Could you check a few things on this model? Use its own coordinates, in mm. Face numbers are marked on the shaded views. A direction names the side the tool comes from. Coordinates: 2 decimals unless noted, no trailing zeros. Loops run counter-clockwise (first coordinate to the right, second up) from the corner with the lowest first, then second, coordinate; pieces in that order, holes last. Notation, with made-up numbers: (-10.5, 2) - (3.5, 2) arc R15 ccw to (3.5, 22) - close; hole circle Ø8 at (-39, 34). An arc over 180 degrees is marked (long way). One line per item, written item: value. Start each with the question number.
(1) If I drill on line 1 along Y through (x, z) = (0, 25.75); line 2 along Z through (x, y) = (-3.75, -5); line 3 along Z through (x, y) = (1.75, 0.5), over which ranges is the centre line in solid material (lowest first)? Write a range as from..to.
(2) If we section it at B-B on x = 0: Write out the boundary of the cut face in (y, z), then the cut area to 3 significant figures.
(3) If we section it at A-A on y = 0: Write out the boundary of the cut face in (x, z).
(4) If we mould it in two halves opening along X, with no side actions, what happens to the marked faces 1, 2 and 3? For each: pulls with the +X half, pulls with the -X half, needs draft (parallel to the pull), parting line crosses it, or undercut.
(5) I'm going to push flat-ended pins straight in: P1, Ø1.5, axis at y = 2, z = 23, coming from the -X side; P2, Ø5, axis at x = -6.5, z = 26.5, coming from the -Y side; P3, Ø4, axis at y = 0, z = 28, coming from the +X side. Where does each tip first touch, or does it pass through?
(6) On a 3-axis mill with a long thin cutter (end or side, diameter ignored), from which of +Z, -Z, +X, -X, +Y, -Y can I reach the whole of each face in a straight line? I mean the marked faces 4, 5 and 6. Say none if no direction works.
(7) If we section it at C-C on z = 5.75: Write out the boundary of the cut face in (x, y).
(8) If we section it at D-D on z = 18.75: Write out the boundary of the cut face in (x, y).
Autodesk Inventor part; units mm, degrees
ref_plane "YZ Plane" through (0, 0, 0) normal (1, 0, 0) x (0, 1, 0)
ref_plane "XZ Plane" through (0, 0, 0) normal (0, 1, 0) x (-1, 0, 0)
ref_plane "XY Plane" through (0, 0, 0) normal (0, 0, 1) x (1, 0, 0)
sketch "Sketch1" plane through (0, 0, 0) normal (0, 0, 1) x (1, 0, 0)
  circle A0 centre (0, 0) radius 9
  dimension "d0" = 18
extrude "Extrusion1" add sketch "Sketch1" along normal blind 10
chamfer "Chamfer1" distance 0.5 angle 45 1 edges at (-9, 0, 0)
sketch "Sketch2" plane through (0, 0, 0) normal (0, 0, -1) x (-1, 0, 0)
  circle A0 centre (0, 0) radius 2.75
  dimension "d6" = 5.5
extrude "Extrusion2" cut sketch "Sketch2" against normal blind 5
sketch "Sketch3" plane through (0, 0, 10) normal (0, 0, 1) x (1, 0, 0)
  circle A0 centre (0, 0) radius 5
  dimension "d9" = 10
extrude "Extrusion3" add sketch "Sketch3" along normal blind 20
sketch "Sketch4" plane through (0, 0, 30) normal (0, 0, 1) x (1, 0, 0)
  arc A0 (-1.1, -1.7889) -> (-1.1, 1.7889) centre (0, 0) ccw
  line L0 (-1.1, 1.7889) -> (-1.1, -1.7889)
  dimension "d12" = 4.2
  dimension "d13" = 1.1
extrude "Extrusion4" cut sketch "Sketch4" against normal blind 7
properties part number "MotorFlyWheel"
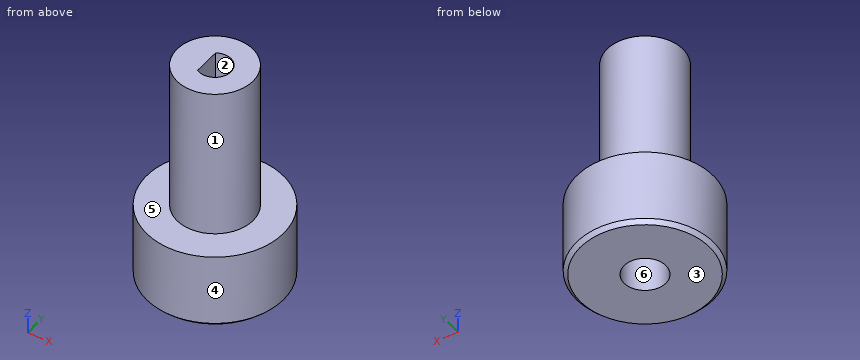
Values:
1. line 1: y = -5..-2.1, 2.1..5
1. line 2: z = 0..10
1. line 3: z = 5..23
2. outline: (-9, 0.5) - (-8.5, 0) - (-2.75, 0) - (-2.75, 5) - (2.75, 5) - (2.75, 0) - (8.5, 0) - (9, 0.5) - (9, 10) - (5, 10) - (5, 30) - (2.1, 30) - (2.1, 23) - (-2.1, 23) - (-2.1, 30) - (-5, 30) - (-5, 10) - (-9, 10) - close
2. area: 323 mm2
3. outline: (-9, 0.5) - (-8.5, 0) - (-2.75, 0) - (-2.75, 5) - (2.75, 5) - (2.75, 0) - (8.5, 0) - (9, 0.5) - (9, 10) - (5, 10) - (5, 30) - (2.1, 30) - (2.1, 23) - (-1.1, 23) - (-1.1, 30) - (-5, 30) - (-5, 10) - (-9, 10) - close
4. face 1: parting line crosses it
4. face 2: undercut
4. face 3: needs draft
5. P1: stops at x = -4.84
5. P2: stops at y = -3
5. P3: stops at x = 5
6. face 4: +Z, -Z
6. face 5: +Z
6. face 6: -Z
7. outline: circle Ø18 at (0, 0)
8. outline: circle Ø10 at (0, 0)
